Read the model definition and answer for the solid it produces. Units are mm, in the model's axes. Face numbers are marked on the shaded views. A direction names the side the tool comes from. Round coordinates to 2 decimals unless told otherwise and drop trailing zeros. Write each loop counter-clockwise with the first axis right and the second up, starting at its lowest first coordinate (ties: lowest second). Pieces come first, ordered by that corner, then holes. Notation, with made-up numbers: (66, 29.25) - (84, 29.25) arc R7 ccw to (84, 36.25) - close; hole circle Ø11 at (25.25, 12.25). An arc over 180 degrees is marked (long way). Answer as CSV lines item,"result". Start each with the question number.
1) Find section B-B on y = 47.5. Determine the outline of the cut face in (x, z).
2) Each of these flat-tipped pins is pushed along its axis until it touches: pin 1 (5 mm diameter, centred on x = -23, z = -82.5, fed in from -Y); pin 2 (2 mm diameter, centred on y = 36.5, z = -92.5, fed in from -X); pin 3 (9.5 mm diameter, centred on x = 4.5, y = 29, fed in from -Z). Where does it stop, or does it pass through?
3) Find section C-C on z = -20. Determine the outline of the cut face in (x, y), then the cut area to 3 significant figures.
4) Consider line 1 along Z through (x, y) = (-13, 34); line 2 along Z through (x, y) = (5, 47); line 3 along X through (y, z) = (4.5, -9). Determine where each line is inside the solid, lowest interval first.
5) Which of the six approach directions +Z, -Z, +X, -X, +Y, -Y give full straight-line access (tool end or side, diameter ignored) to the marked faces 1, 2 and 3?
6) Find section D-D on x = 7. Determine the outline of the cut face in (y, z).
7) Find section A-A on y = 36.5. Determine the outline of the cut face in (x, z), then the cut area to 3 significant figures.
from build123d import *

# Parameters (mm, degrees)
BOSS_EXTRUDE1_DEPTH = 9.5
BOSS_EXTRUDE2_DEPTH = 103


with BuildPart() as part:
    # Sketch1 → Boss-Extrude1 (new body)
    with BuildSketch(Plane.XY):
        Polygon((0, 0), (-11.5, 65.219740926), (11.5, 65.219740926), align=None)
    extrude(amount=-BOSS_EXTRUDE1_DEPTH)

    # Sketch2 → Boss-Extrude2 (add)
    with BuildSketch(Plane(origin=(0, 0, -9.5), x_dir=(-1, 0, 0), z_dir=(0, 0, -1))):
        Polygon((-11.5, 65.219740926), (36.5, 65.219740926), (12.5, 33.219740926), align=None)
    extrude(amount=BOSS_EXTRUDE2_DEPTH)


solid = part.part
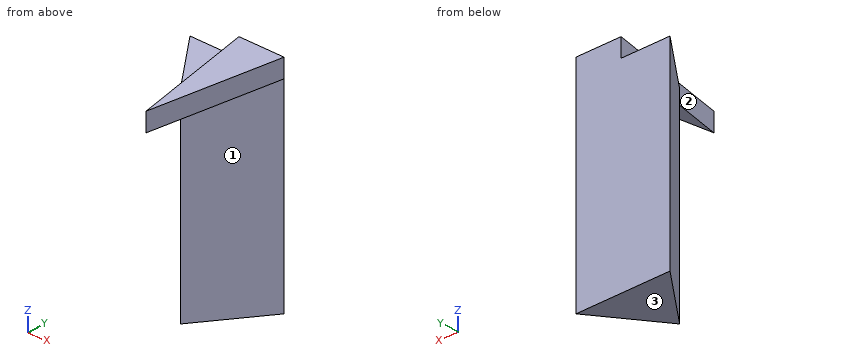
Check values:
1,outline,"(-23.21, -112.5) - (-1.79, -112.5) - (-1.79, -9.5) - (8.38, -9.5) - (8.38, 0) - (-8.38, 0) - (-8.38, -9.5) - (-23.21, -9.5) - close"
2,pin 1,"stops at y = 43.89"
2,pin 2,"stops at x = -15.71"
2,pin 3,"stops at z = -9.5"
3,outline,"(-36.5, 65.22) - (-12.5, 33.22) - (11.5, 65.22) - close"
3,area,"768 mm^2"
4,line 1,"z = -112.5 to -9.5"
4,line 2,"z = -9.5 to 0"
4,line 3,"x = -0.79 to 0.79"
5,face 1,"-Z, +X, -Y"
5,face 2,"+Z, -X, -Y"
5,face 3,"-Z, +X, -X, +Y, -Y"
6,outline,"(39.7, -9.5) - (59.22, -9.5) - (59.22, -112.5) - (65.22, -112.5) - (65.22, 0) - (39.7, 0) - close"
7,outline,"(-14.96, -112.5) - (-10.04, -112.5) - (-10.04, -9.5) - (-14.96, -9.5) - close; (-6.44, -9.5) - (6.44, -9.5) - (6.44, 0) - (-6.44, 0) - close"
7,area,"629 mm^2"
